```python
from build123d import *

# Parameters (mm, degrees)
SKETCH1_W           = 29.69848481
SKETCH1_H           = 29.69848481
SKETCH1_R           = 5
SKETCH1_R_2         = 1.6
BOSS_EXTRUDE1_DEPTH = 2.5
CUT_EXTRUDE1_DEPTH  = 22.148285983
FILLET3_R           = 1
CHAMFER1_SIZE       = 1.5


with BuildPart() as part:
    # Sketch1 → Boss-Extrude1 (new body)
    with BuildSketch(Plane(origin=(0, 0, 0), x_dir=(1, 0, 0), z_dir=(0, 1, 0))):
        Rectangle(SKETCH1_W, SKETCH1_H)
        with Locations(Location((0, 0, 0), (0, 0, 270))):
            Circle(SKETCH1_R, mode=Mode.SUBTRACT)
        with Locations(Location((-5.656854249, 5.656854249, 0), (0, 0, 270))):
            Circle(SKETCH1_R_2, mode=Mode.SUBTRACT)
        with Locations(Location((5.656854249, -5.656854249, 0), (0, 0, 270))):
            Circle(SKETCH1_R_2, mode=Mode.SUBTRACT)
        with Locations(Location((-6.717514421, -6.717514421, 0), (0, 0, 270))):
            Circle(SKETCH1_R_2, mode=Mode.SUBTRACT)
        with Locations(Location((6.717514421, 6.717514421, 0), (0, 0, 270))):
            Circle(SKETCH1_R_2, mode=Mode.SUBTRACT)
        with Locations(Location((-11.66726189, -11.66726189, 0), (0, 0, 270))):
            Circle(SKETCH1_R_2, mode=Mode.SUBTRACT)
        with Locations(Location((-11.66726189, 11.66726189, 0), (0, 0, 270))):
            Circle(SKETCH1_R_2, mode=Mode.SUBTRACT)
        with Locations(Location((11.66726189, 11.66726189, 0), (0, 0, 270))):
            Circle(SKETCH1_R_2, mode=Mode.SUBTRACT)
        with Locations(Location((11.66726189, -11.66726189, 0), (0, 0, 270))):
            Circle(SKETCH1_R_2, mode=Mode.SUBTRACT)
    extrude(amount=BOSS_EXTRUDE1_DEPTH)

    # Sketch2 → Cut-Extrude1 (cut, through all)
    with BuildSketch(Plane(origin=(0, 2.5, 0), x_dir=(1, 0, 0), z_dir=(0, 1, 0))):
        with BuildLine():
            Line((-9.899494937, 4.949747468), (-14.849242405, 9.899494937))
            Line((-14.849242405, 9.899494937), (-14.849242405, -9.899494937))
            Line((-14.849242405, -9.899494937), (-9.899494937, -4.949747468))
            ThreePointArc((-9.899494937, -4.949747468), (-7.849242405, 0), (-9.899494937, 4.949747468))
        make_face()
        with BuildLine():
            Line((9.899494937, 14.849242405), (-9.899494937, 14.849242405))
            Line((-9.899494937, 14.849242405), (-4.949747468, 9.899494937))
            ThreePointArc((-4.949747468, 9.899494937), (0, 7.849242405), (4.949747468, 9.899494937))
            Line((4.949747468, 9.899494937), (9.899494937, 14.849242405))
        make_face()
        with BuildLine():
            Line((14.849242405, -9.899494937), (14.849242405, 9.899494937))
            Line((14.849242405, 9.899494937), (9.899494937, 4.949747468))
            ThreePointArc((9.899494937, 4.949747468), (7.849242405, 0), (9.899494937, -4.949747468))
            Line((9.899494937, -4.949747468), (14.849242405, -9.899494937))
        make_face()
        with BuildLine():
            Line((-9.899494937, -14.849242405), (9.899494937, -14.849242405))
            Line((9.899494937, -14.849242405), (4.949747468, -9.899494937))
            ThreePointArc((4.949747468, -9.899494937), (0, -7.849242405), (-4.949747468, -9.899494937))
            Line((-4.949747468, -9.899494937), (-9.899494937, -14.849242405))
        make_face()
    extrude(amount=-CUT_EXTRUDE1_DEPTH, mode=Mode.SUBTRACT)

    # Fillet3
    fillet3_edges = [part.edges().sort_by_distance(p)[0] for p in [
        (14.849242405, 1.25, -9.899494937),
        (14.849242405, 1.25, 9.899494937),
        (14.849242405, 1.25, 14.849242405),
        (-14.849242405, 1.25, 14.849242405),
        (-14.849242405, 1.25, -14.849242405),
        (-9.899494937, 1.25, -14.849242405),
        (9.899494937, 1.25, -14.849242405),
        (14.849242405, 1.25, -14.849242405),
        (9.899494937, 1.25, 14.849242405),
        (-9.899494937, 1.25, 14.849242405),
        (-14.849242405, 1.25, 9.899494937),
        (-14.849242405, 1.25, -9.899494937),
    ]]
    fillet(fillet3_edges, radius=FILLET3_R)

    # Chamfer1
    # the kernel refuses this chamfer: 1.5 mm, written as the material it takes off along each edge
    with BuildSketch(Plane(origin=(-5.656854249, 2.5, -5.656854249), x_dir=(0, 0, 1), z_dir=(-1, 0, 0))) as chamfer1_piece_1:
        Polygon((1.6 + CHAMFER1_SIZE, 0), (1.6, -CHAMFER1_SIZE), (1.6, 0), align=None)
    revolve(axis=Axis((-5.656854249, 2.5, -5.656854249), (0, 1, 0)), mode=Mode.SUBTRACT)
    with BuildSketch(Plane(origin=(5.656854249, 2.5, 5.656854249), x_dir=(0, 0, 1), z_dir=(-1, 0, 0))) as chamfer1_piece_2:
        Polygon((1.6 + CHAMFER1_SIZE, 0), (1.6, -CHAMFER1_SIZE), (1.6, 0), align=None)
    revolve(axis=Axis((5.656854249, 2.5, 5.656854249), (0, 1, 0)), mode=Mode.SUBTRACT)
    with BuildSketch(Plane(origin=(-6.717514421, 2.5, 6.717514421), x_dir=(0, 0, 1), z_dir=(-1, 0, 0))) as chamfer1_piece_3:
        Polygon((1.6 + CHAMFER1_SIZE, 0), (1.6, -CHAMFER1_SIZE), (1.6, 0), align=None)
    revolve(axis=Axis((-6.717514421, 2.5, 6.717514421), (0, 1, 0)), mode=Mode.SUBTRACT)
    with BuildSketch(Plane(origin=(6.717514421, 2.5, -6.717514421), x_dir=(0, 0, 1), z_dir=(-1, 0, 0))) as chamfer1_piece_4:
        Polygon((1.6 + CHAMFER1_SIZE, 0), (1.6, -CHAMFER1_SIZE), (1.6, 0), align=None)
    revolve(axis=Axis((6.717514421, 2.5, -6.717514421), (0, 1, 0)), mode=Mode.SUBTRACT)
    with BuildSketch(Plane(origin=(-11.66726189, 0, 11.66726189), x_dir=(0, 0, 1), z_dir=(-1, 0, 0))) as chamfer1_piece_5:
        Polygon((1.6 + CHAMFER1_SIZE, 0), (1.6, CHAMFER1_SIZE), (1.6, 0), align=None)
    revolve(axis=Axis((-11.66726189, 0, 11.66726189), (0, 1, 0)), mode=Mode.SUBTRACT)
    with BuildSketch(Plane(origin=(-11.66726189, 0, -11.66726189), x_dir=(0, 0, 1), z_dir=(-1, 0, 0))) as chamfer1_piece_6:
        Polygon((1.6 + CHAMFER1_SIZE, 0), (1.6, CHAMFER1_SIZE), (1.6, 0), align=None)
    revolve(axis=Axis((-11.66726189, 0, -11.66726189), (0, 1, 0)), mode=Mode.SUBTRACT)
    with BuildSketch(Plane(origin=(11.66726189, 0, -11.66726189), x_dir=(0, 0, 1), z_dir=(-1, 0, 0))) as chamfer1_piece_7:
        Polygon((1.6 + CHAMFER1_SIZE, 0), (1.6, CHAMFER1_SIZE), (1.6, 0), align=None)
    revolve(axis=Axis((11.66726189, 0, -11.66726189), (0, 1, 0)), mode=Mode.SUBTRACT)
    with BuildSketch(Plane(origin=(11.66726189, 0, 11.66726189), x_dir=(0, 0, 1), z_dir=(-1, 0, 0))) as chamfer1_piece_8:
        Polygon((1.6 + CHAMFER1_SIZE, 0), (1.6, CHAMFER1_SIZE), (1.6, 0), align=None)
    revolve(axis=Axis((11.66726189, 0, 11.66726189), (0, 1, 0)), mode=Mode.SUBTRACT)


solid = part.part
```
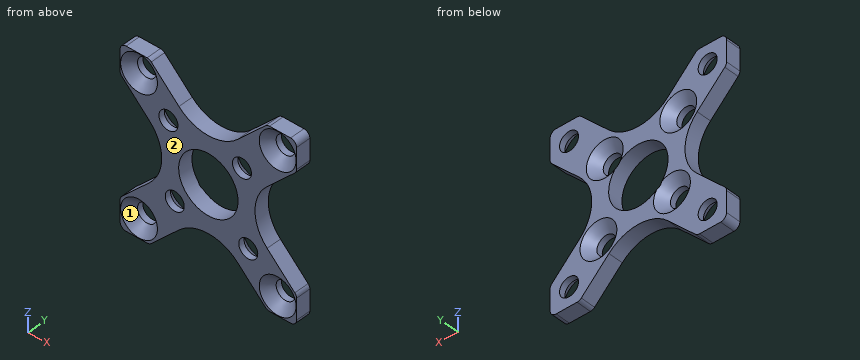
Part model, mm, in its own coordinate system. Face numbers are marked on the shaded views. Round coordinates to 2 decimals unless told otherwise and drop trailing zeros. Write each loop counter-clockwise with the first axis right and the second up, starting at its lowest first coordinate (ties: lowest second). Pieces come first, ordered by that corner, then holes. Notation, with made-up numbers: M -10,-9 L 42,-9 A37 cw 42,30 Z; hole C 85,-39.75 d5. An arc over 180 degrees is marked long. Answer as CSV lines item,"result". Start each with the question number.
1) Mould opens along X. For the marked faces 1 and 2 say: +X half, -X half, draft (parallel to the pull), parting line (faces both ways), or undercut.
2) Band-saw the part on A-A (z = 0). List the corners of the cut face in (x, y).
3) Band-saw the part on C-C (x = -6.25). Count the separate pieces of the cut face and the enclosed holes in it, then the cut area to 4 significant figures.
4) Drop a flat-ended pin along its axis: pin 1 (1 mm diameter, centred on y = 0.5, z = 5.5, fed in from -X). Give the stop position or say it passes through.
5) Band-saw the part on B-B (x = 0). List the corners of the cut face in (y, z), then the cut area to 3 significant figures.
6) Drill centre lines: L1, parallel to X at y = 0.1, z = 9; L2, parallel to X at y = 1.6, z = -5.75; L3, parallel to Z at x = -13, y = 0.7. Where is each one in solid material? Low to high.
Worked out:
1,face 1,"undercut"
1,face 2,"draft"
2,outline,"M -7.85,0 L -5,0 L -5,2.5 L -7.85,2.5 Z; M 5,0 L 7.85,0 L 7.85,2.5 L 5,2.5 Z"
3,separate pieces,"3"
3,enclosed holes,"0"
3,area,"36.25 mm²"
4,pin 1,"x = -10.95"
5,outline,"M 0,-7.85 L 2.5,-7.85 L 2.5,-5 L 0,-5 Z; M 0,5 L 2.5,5 L 2.5,7.85 L 0,7.85 Z"
5,area,"14.2 mm²"
6,L1,"-13.95 to -13.04, -10.29 to -3.85, 3.85 to 10.29, 13.04 to 13.95"
6,L2,"-10.7 to -7.85, -3.46 to 4.74, 8.69 to 10.7"
6,L3,"-14.85 to -13.66, -9.67 to -8.05, 8.05 to 9.67, 13.66 to 14.85"
